from build123d import *

# Parameters (mm, degrees)
SKETCH1_R           = 1.5
SKETCH1_R_2         = 1.45
BOSS_EXTRUDE1_DEPTH = 2
SKETCH_1_R          = 1.45
SKETCH_1_R_2        = 1.5
EXTRUDE_1_DEPTH     = 2
EXTRUDE_2_DEPTH     = 2
FILLET1_R           = 1


with BuildPart() as part:
    # Sketch1 → Boss-Extrude1 (new body)
    with BuildSketch(Plane(origin=(0, 0, 0), x_dir=(1, 0, 0), z_dir=(0, 1, 0))):
        with BuildLine():
            Line((-21.192961085, -132.078714637), (-21.192961085, -166.219718768))
            Line((-21.192961085, -166.219718768), (-14.185358568, -176.236618152))
            ThreePointArc((-14.185358568, -176.236618152), (-13.513427934, -177.60024794), (-13.282330236, -179.10276943))
            Line((-13.282330236, -179.10276943), (-13.282330236, -193.470906367))
            ThreePointArc((-13.282330236, -193.470906367), (-14.74679633, -197.006440273), (-18.282330236, -198.470906367))
            Line((-18.282330236, -198.470906367), (-21.77517331, -198.470906367))
            Line((-21.77517331, -198.470906367), (-31.192961085, -198.470906367))
            ThreePointArc((-31.192961085, -198.470906367), (-34.728494991, -197.006440273), (-36.192961085, -193.470906367))
            Line((-36.192961085, -193.470906367), (-36.192961085, -90.830339434))
            ThreePointArc((-36.192961085, -90.830339434), (-34.909297601, -87.485366654), (-31.717423925, -85.857921639))
            Line((-31.717423925, -85.857921639), (-19.324348326, -84.550769285))
            Line((-19.324348326, -84.550769285), (-12.49642386, -84.082177413))
            Line((-12.49642386, -84.082177413), (3.10357614, -84.082177413))
            Line((3.10357614, -84.082177413), (3.307038915, -84.078714637))
            Line((3.307038915, -84.078714637), (3.307038915, -109.367146032))
            ThreePointArc((3.307038915, -109.367146032), (-2.41677201, -116.354903712), (-9.40452969, -122.078714637))
            Line((-9.40452969, -122.078714637), (-14.349438262, -125.02189202))
            Line((-14.349438262, -125.02189202), (-21.192961085, -126.237284003))
            Line((-21.192961085, -126.237284003), (-21.192961085, -132.078714637))
        make_face()
        with Locations(Location((-18.919157596, -192.204354167, 0), (0, 0, 270))):
            Circle(SKETCH1_R, mode=Mode.SUBTRACT)
        with Locations(Location((-18.919157596, -178.204354167, 0), (0, 0, 270))):
            Circle(SKETCH1_R, mode=Mode.SUBTRACT)
        with Locations(Location((-31.717423925, -178.204354167, 0), (0, 0, 270))):
            Circle(SKETCH1_R, mode=Mode.SUBTRACT)
        with Locations(Location((-31.717423925, -192.204354167, 0), (0, 0, 270))):
            Circle(SKETCH1_R, mode=Mode.SUBTRACT)
        with Locations(Location((-29.287619577, -102.069022085, 0), (0, 0, 270))):
            Circle(SKETCH1_R, mode=Mode.SUBTRACT)
        with Locations(Location((-16.702653636, -89.484056145, 0), (0, 0, 270))):
            Circle(SKETCH1_R, mode=Mode.SUBTRACT)
        with Locations(Location((1.158345759, -107.272976806, 0), (0, 0, 270))):
            Circle(SKETCH1_R_2, mode=Mode.SUBTRACT)
        with Locations(Location((-4.499501528, -114.272174194, 0), (0, 0, 270))):
            Circle(SKETCH1_R_2, mode=Mode.SUBTRACT)
        with Locations(Location((-11.498698916, -119.930021481, 0), (0, 0, 270))):
            Circle(SKETCH1_R_2, mode=Mode.SUBTRACT)
        with Locations(Location((-29.287619577, -127.462503818, 0), (0, 0, 270))):
            Circle(SKETCH1_R, mode=Mode.SUBTRACT)
        with Locations(Location((-29.287619577, -143.302559608, 0), (0, 0, 270))):
            Circle(SKETCH1_R, mode=Mode.SUBTRACT)
        with Locations(Location((-31.442028499, -91.953708305, 0), (0, 0, 270))):
            Circle(SKETCH1_R, mode=Mode.SUBTRACT)
        with BuildLine():
            Line((-3.683855698, -92.504640443), (-7.556212498, -91.467045565))
            ThreePointArc((-7.556212498, -91.467045565), (-9.011313317, -91.632215687), (-9.963793597, -92.744591918))
            ThreePointArc((-9.963793597, -92.744591918), (-16.148276393, -102.623399329), (-26.027083804, -108.807882125))
            ThreePointArc((-26.027083804, -108.807882125), (-27.139460035, -109.760362404), (-27.304630157, -111.215463223))
            Line((-27.304630157, -111.215463223), (-26.267035279, -115.087820024))
            ThreePointArc((-26.267035279, -115.087820024), (-25.280541686, -116.332651264), (-23.697816809, -116.465904366))
            ThreePointArc((-23.697816809, -116.465904366), (-10.491422144, -108.280253578), (-2.305771356, -95.073858913))
            ThreePointArc((-2.305771356, -95.073858913), (-2.439024458, -93.491134036), (-3.683855698, -92.504640443))
        make_face(mode=Mode.SUBTRACT)
    extrude(amount=BOSS_EXTRUDE1_DEPTH)

    # 草图1 → 凸台-拉伸1 (add)
    with BuildSketch(Plane.XZ):
        with BuildLine():
            Line((-12.69642386, 84.082177413), (-12.69642386, 58.793746018))
            ThreePointArc((-12.69642386, 58.793746018), (-6.972612935, 51.805988338), (0.015144745, 46.082177413))
            Line((0.015144745, 46.082177413), (25.30357614, 46.082177413))
            Line((25.30357614, 46.082177413), (50.592007535, 46.082177413))
            ThreePointArc((50.592007535, 46.082177413), (57.579765215, 51.805988338), (63.30357614, 58.793746018))
            Line((63.30357614, 58.793746018), (63.30357614, 84.078714637))
            Line((63.30357614, 84.078714637), (47.168942899, 84.078714637))
            Line((47.168942899, 84.078714637), (43.263289357, 80.173061094))
            ThreePointArc((43.263289357, 80.173061094), (44.35454376, 77.612712957), (41.794195623, 78.70396736))
            Line((41.794195623, 78.70396736), (40.962688124, 77.872459862))
            ThreePointArc((40.962688124, 77.872459862), (37.21418877, 72.168102006), (31.509830915, 68.419602653))
            ThreePointArc((31.509830915, 68.419602653), (29.563736563, 67.782199069), (27.554675458, 67.385664037))
            Line((27.554675458, 67.385664037), (23.052476821, 67.389126813))
            ThreePointArc((23.052476821, 67.389126813), (21.043415716, 67.785661845), (19.097321364, 68.423065428))
            ThreePointArc((19.097321364, 68.423065428), (13.392963509, 72.171564782), (9.644464155, 77.875922638))
            Line((9.644464155, 77.875922638), (8.812956657, 78.707430136))
            ThreePointArc((8.812956657, 78.707430136), (6.25260852, 77.616175733), (7.343862923, 80.17652387))
            Line((7.343862923, 80.17652387), (3.43820938, 84.082177413))
            Line((3.43820938, 84.082177413), (-12.69642386, 84.082177413))
        make_face()
        with Locations(Location((61.154882984, 60.887915244, 0), (0, 0, 90))):
            Circle(SKETCH_1_R, mode=Mode.SUBTRACT)
        with Locations(Location((55.497035696, 53.888717856, 0), (0, 0, 90))):
            Circle(SKETCH_1_R, mode=Mode.SUBTRACT)
        with Locations(Location((48.497838309, 48.230870569, 0), (0, 0, 90))):
            Circle(SKETCH_1_R, mode=Mode.SUBTRACT)
        with Locations(Location((30.708917648, 66.091869964, 0), (0, 0, 90))):
            Circle(SKETCH_1_R_2, mode=Mode.SUBTRACT)
        with Locations(Location((2.109313971, 48.230870569, 0), (0, 0, 90))):
            Circle(SKETCH_1_R, mode=Mode.SUBTRACT)
        with Locations(Location((-4.889883417, 53.888717856, 0), (0, 0, 90))):
            Circle(SKETCH_1_R, mode=Mode.SUBTRACT)
        with Locations(Location((-10.547730705, 60.887915244, 0), (0, 0, 90))):
            Circle(SKETCH_1_R, mode=Mode.SUBTRACT)
        with Locations(Location((19.898234632, 66.091869964, 0), (0, 0, 90))):
            Circle(SKETCH_1_R_2, mode=Mode.SUBTRACT)
        with BuildLine():
            Line((52.440324726, 76.693846485), (56.312681527, 75.656251607))
            ThreePointArc((56.312681527, 75.656251607), (57.557512766, 74.669758014), (57.690765869, 73.087033137))
            ThreePointArc((57.690765869, 73.087033137), (49.505115081, 59.880638472), (36.298720415, 51.694987684))
            ThreePointArc((36.298720415, 51.694987684), (34.715995538, 51.828240786), (33.729501945, 53.073072026))
            Line((33.729501945, 53.073072026), (32.691907068, 56.945428827))
            ThreePointArc((32.691907068, 56.945428827), (32.857077189, 58.400529646), (33.96945342, 59.353009925))
            ThreePointArc((33.96945342, 59.353009925), (43.848260831, 65.537492721), (50.032743627, 75.416300132))
            ThreePointArc((50.032743627, 75.416300132), (50.985223907, 76.528676363), (52.440324726, 76.693846485))
        make_face(mode=Mode.SUBTRACT)
        with BuildLine():
            Line((17.915245212, 56.945428827), (16.877650334, 53.073072026))
            ThreePointArc((16.877650334, 53.073072026), (15.891156741, 51.828240786), (14.308431864, 51.694987684))
            ThreePointArc((14.308431864, 51.694987684), (1.102037199, 59.880638472), (-7.083613589, 73.087033137))
            ThreePointArc((-7.083613589, 73.087033137), (-6.950360487, 74.669758014), (-5.705529247, 75.656251607))
            Line((-5.705529247, 75.656251607), (-1.833172447, 76.693846485))
            ThreePointArc((-1.833172447, 76.693846485), (-0.378071628, 76.528676363), (0.574408652, 75.416300132))
            ThreePointArc((0.574408652, 75.416300132), (6.758891448, 65.537492721), (16.637698859, 59.353009925))
            ThreePointArc((16.637698859, 59.353009925), (17.75007509, 58.400529646), (17.915245212, 56.945428827))
        make_face(mode=Mode.SUBTRACT)
    extrude(amount=-EXTRUDE_1_DEPTH)

    # 草图2 → 凸台-拉伸2 (add)
    with BuildSketch(Plane.XZ):
        with BuildLine():
            Line((-12.443677961, 84.250317512), (-17.409343258, 84.591104879))
            ThreePointArc((-17.409343258, 84.591104879), (-14.024568956, 81.869997058), (-12.443677961, 77.825011457))
            Line((-12.443677961, 77.825011457), (-12.443677961, 84.250317512))
        make_face()
    extrude(amount=-EXTRUDE_2_DEPTH)

    # Fillet1
    fillet1_edges = [part.edges().sort_by_distance(p)[0] for p in [
        (-21.192961085, 1, 126.237284003),
    ]]
    fillet(fillet1_edges, radius=FILLET1_R)


solid = part.part
Design review of the part built by this model. Coordinates are the model's own, in mm. A direction names the side the tool comes from. Give positions to 0.01 mm unless a question says otherwise; leave off trailing zeros. Loops run counter-clockwise (first coordinate to the right, second up) from the corner with the lowest first, then second, coordinate; pieces in that order, holes last. Notation, with made-up numbers: M 80.5,41.25 L 122.5,41.25 A30 cw 122.5,66.25 Z; hole C -10,72 d4. An arc over 180 degrees is marked long. One line per question, with ' | ' between items. Start each with the question number.
1. Insertion check: P1, Ø2.5, axis at x = -31.72, z = 178.2, coming from the -Y side; P2, Ø3.5, axis at x = 61.15, z = 60.89, coming from the -Y side; P3, Ø0.6, axis at y = 0.5, z = 73.5, coming from the -X side. Each pin has a flat end and moves straight along its axis. Give the tip position at first contact, or say it passes through.
2. Add section D-D (x = 25.5). Write out the cut boundary in (y, z).
3. To check wall thickness, follow L1, parallel to Z at x = 48, y = 1.8; L2, parallel to X at y = 0.9, z = 65; L3, parallel to X at y = 1.25, z = 114. State the ranges of each line that lie inside material, in increasing order.
4. Add section B-B (z = 139.5). Write out the cut boundary in (x, y).
5. For faces 1 (the face through (-14.32, 0.99, 82.25)), 2 (the face through (45.24, 0.99, 82.15)), 3 (the face through (49.66, 0.986, 60.036)), 4 (the face through (-17.738, 0.986, 171.158)), list the 3-axis set-ups (+Z, -Z, +X, -X, +Y, -Y) from which the entire face can be reached by the end or side of a thin tool; tool diameter is ignored.
6. Add section C-C (y = 0.9). Give the number of separate pieces and of enclosed holes in the cut face, plus the area to 3 significant figures.
7. Add section A-A (z = 82). Write out the cut boundary in (x, y).
8. The part is to be moulded in two halves that separate along Z. For faces 5 (the face through (-19.49, 0.99, 193.59)), 6 (the face through (-2.33, 0.99, 116.27)), 7 (the face through (-7.062, 0.986, 51.896)), 8 (the face through (2.665, 0.986, 49.57)), say which applies: released by +Z, released by -Z, zero draft, split by the parting line, or undercut.
Worked out:
1) P1: passes through | P2: stops at y = 0 | P3: stops at x = -12.7
2) outline: M 0,46.08 L 2,46.08 L 2,67.39 L 0,67.39 Z
3) L1: z = 46.08 to 46.87, 49.59 to 58.46, 70.96 to 84.08 | L2: x = -12.7 to -3.1, 7.31 to 18.87, 20.93 to 29.68, 31.74 to 43.29, 53.71 to 63.3 | L3: x = -36.19 to -26.56, -18.09 to -5.92, -3.08 to -0.22
4) outline: M -36.19,0 L -21.19,0 L -21.19,2 L -36.19,2 Z
5) face 1: -Z, -X, +Y, -Y | face 2: +Z, +Y, -Y | face 3: +Y, -Y | face 4: +X, +Y, -Y
6) separate pieces: 1 | enclosed holes: 23 | area: 4,170 mm²
7) outline: M -14.12,0 L 5.52,0 L 5.52,2 L -14.12,2 Z; M 45.09,0 L 63.3,0 L 63.3,2 L 45.09,2 Z
8) face 5: undercut | face 6: released by +Z | face 7: released by -Z | face 8: undercut
